Model file for the job. Use its own axes, mm. A direction names the side the tool comes from. Coordinates: 2 decimals unless noted, no trailing zeros. Write each loop counter-clockwise with the first axis right and the second up, starting at its lowest first coordinate (ties: lowest second). Pieces come first, ordered by that corner, then holes. Notation, with made-up numbers: M 5,49 L 59,49 A4 cw 59,56 Z; hole C 58.5,-38 d5. An arc over 180 degrees is marked long. Put each result on its own line as item: value. Start each with the question number.
Q1. Cut at A-A (x = 0). Write the cut outline in (y, z).
Q2. Cut at D-D (x = 3). Write the cut outline in (y, z), then the cut area to 3 significant figures.
Q3. Which spindle directions (+Z, -Z, +X, -X, +Y, -Y) get a long thin tool onto all of the face, cutting with end or side? Do faces 1 (the flat face through (2, 2, 1.6)), 2 (the flat face through (0, -3.975, 1)). Say none if no direction does.
Q4. Drop flat-ended pins along their axis: pin 1 (1 mm diameter, centred on y = 2.5, z = 14.5, fed in from +X); pin 2 (1.5 mm diameter, centred on x = 2, y = 2, fed in from +Z); pin 3 (2 mm diameter, centred on y = -2.5, z = 9.5, fed in from -X). Give the stop position or say it passes through.
Q5. Cut at C-C (y = 2.75). Write the cut outline in (x, z).
Q6. Cut at B-B (z = 9). Write the cut outline in (x, y), then the cut area to 3 significant figures.
Q7. Drill centre lines: line 1 along Z through (x, y) = (0.5, 3.25); line 2 along Y through (x, z) = (0, 13.5); line 3 along Z through (x, y) = (-2.25, 0.5). Where is each one in solid material? Low to high.
```python
from build123d import *

# Parameters (mm, degrees)
F1_DEPTH = 1.6002
F2_R     = 2.3622
F3_DEPTH = 15.875
F4_SIZE  = 0.381


with BuildPart() as f1:
    # F0 (on Top) → F1 (new body)
    with BuildSketch(Plane.XY):
        Polygon((2.284306, 3.9751), (-2.284306, 3.9751), (-4.5847, 0), (-2.284306, -3.9751), (2.284306, -3.9751), (4.5847, 0), align=None)
    extrude(amount=F1_DEPTH)

    # F2 (on face) → F3 (join)
    with BuildSketch(Plane.XY.offset(1.6002)):
        Circle(F2_R)
    extrude(amount=F3_DEPTH)

    # F4
    f4_edges = [f1.edges().sort_by_distance(p)[0] for p in [
        (-2.3622, 0, 17.4752),
    ]]
    chamfer(f4_edges, length=F4_SIZE)


solid = f1.part
```
Computed values:
1. outline: M -3.98,0 L 3.98,0 L 3.98,1.6 L 2.36,1.6 L 2.36,17.09 L 1.98,17.48 L -1.98,17.48 L -2.36,17.09 L -2.36,1.6 L -3.98,1.6 Z
2. outline: M -2.74,0 L 2.74,0 L 2.74,1.6 L -2.74,1.6 Z
2. area: 8.76 mm2
3. face 1: +Z
3. face 2: +Z, -Z, +X, -X, -Y
4. pin 1: x = 1.26
4. pin 2: z = 17.38
4. pin 3: x = -1.82
5. outline: M -2.99,0 L 2.99,0 L 2.99,1.6 L -2.99,1.6 Z
6. outline: C 0,0 d4.72
6. area: 17.5 mm2
7. line 1: 0 to 1.6
7. line 2: -2.36 to 2.36
7. line 3: 0 to 17.15
